Geometry check sheet. Reference: the model listing, model coordinates, mm. Face numbers are marked on the shaded views. A direction names the side the tool comes from. Coordinates: 2 decimals unless noted, no trailing zeros. Write each loop counter-clockwise with the first axis right and the second up, starting at its lowest first coordinate (ties: lowest second). Pieces come first, ordered by that corner, then holes. Notation, with made-up numbers: (43.25, -12) -> (52.25, -12) arc R22 ccw to (52.25, 2) -> close; hole circle Ø8 at (-36, -26.75). An arc over 180 degrees is marked (long way). Use a Markdown table: item, result.
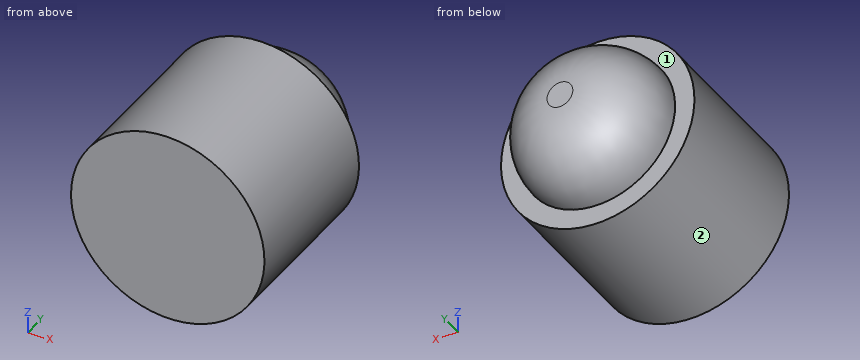
```python
from build123d import *

# Parameters (mm, degrees)
SKETCH1_R           = 15
BOSS_EXTRUDE1_DEPTH = 25
SKETCH2_R           = 12
CUT_EXTRUDE1_DEPTH  = 10
BOSS_EXTRUDE2_START = 20
SKETCH3_R           = 12
BOSS_EXTRUDE2_DEPTH = 20
FILLET1_R           = 10


with BuildPart() as part:
    # Sketch1 → Boss-Extrude1 (new body)
    with BuildSketch(Plane(origin=(0, 0, 0), x_dir=(1, 0, 0), z_dir=(0, 1, 0))):
        with Locations(Location((0, 0, 0), (0, 0, 270))):
            Circle(SKETCH1_R)
    extrude(amount=BOSS_EXTRUDE1_DEPTH)

    # Sketch2 → Cut-Extrude1 (cut)
    with BuildSketch(Plane(origin=(0, 25, 0), x_dir=(1, 0, 0), z_dir=(0, 1, 0))):
        with Locations(Location((0, 0, 0), (0, 0, 270))):
            Circle(SKETCH2_R)
    extrude(amount=-CUT_EXTRUDE1_DEPTH, mode=Mode.SUBTRACT)

    # Sketch3 → Boss-Extrude2 (add)
    with BuildSketch(Plane(origin=(0, 15, 0), x_dir=(1, 0, 0), z_dir=(0, 1, 0)).offset(BOSS_EXTRUDE2_START)):
        with Locations(Location((0, 0, 0), (0, 0, 270))):
            Circle(SKETCH3_R)
    extrude(amount=-BOSS_EXTRUDE2_DEPTH)

    # Fillet1
    fillet1_edges = [part.edges().sort_by_distance(p)[0] for p in [
        (0, 35, -12),
    ]]
    fillet(fillet1_edges, radius=FILLET1_R - 0.0001)  # a hair under: the kernel refuses the full size


solid = part.part
```
Item 1: Depth check by flat-ended pin: P1, Ø4, axis at x = -2, y = 13, coming from the -Z side; P2, Ø10, axis at x = -7.5, y = 14.5, coming from the +Z side; P3, Ø8, axis at y = 31.5, z = -4, coming from the +X side; P4, Ø1, axis at x = -2, z = 10.5, coming from the +Y side. Enter the tip coordinate at first touch or a pass-through.
Answer block:
| item | result |
|---|---|
| P1 | stops at z = -15 |
| P2 | stops at z = 14.79 |
| P3 | stops at x = 11.35 |
| P4 | stops at y = 30.74 |
Item 2: Section check A-A on y = 18.5. Record the boundary of the cut face in (x, z).
Answer block:
| item | result |
|---|---|
| outline | circle Ø30 at (0, 0) |
Item 3: Thickness scan on L1, parallel to Y at x = 12, z = 8.5; L2, parallel to Y at x = 1, z = -2; L3, parallel to X at y = 28, z = -3.5. Record the ranges inside material, lowest first. Write a range as [from, to].
Answer block:
| item | result |
|---|---|
| L1 | y = [0, 25] |
| L2 | y = [0, 35] |
| L3 | x = [-11, 11] |
Item 4: Tool access check on the marked faces 1 and 2. Record the directions out of +Z, -Z, +X, -X, +Y, -Y that give a thin tool (end or side, any length) a straight path to the whole face; none if there is none.
Answer block:
| item | result |
|---|---|
| face 1 | +Y |
| face 2 | +Y, -Y |
